The drawing under review shows one solid part. Ordinate dimensions are in mm from its lowest x, y, z. A direction names the side the tool comes from. Give positions to 0.01 mm unless a question says otherwise; leave off trailing zeros. Order: outer loops, then holes, each group sorted by start corner. A loop starts at its lowest first (then second) coordinate and runs counter-clockwise, first axis right, second up. Notation, with made-up numbers: (42, 45.25) -> (46, 45.25) arc R25 ccw to (46, 74.25) -> close; hole circle Ø8 at (52.5, 58.25). An arc over 180 degrees is marked (long way). Use a Markdown table: item, result. Add a question column.
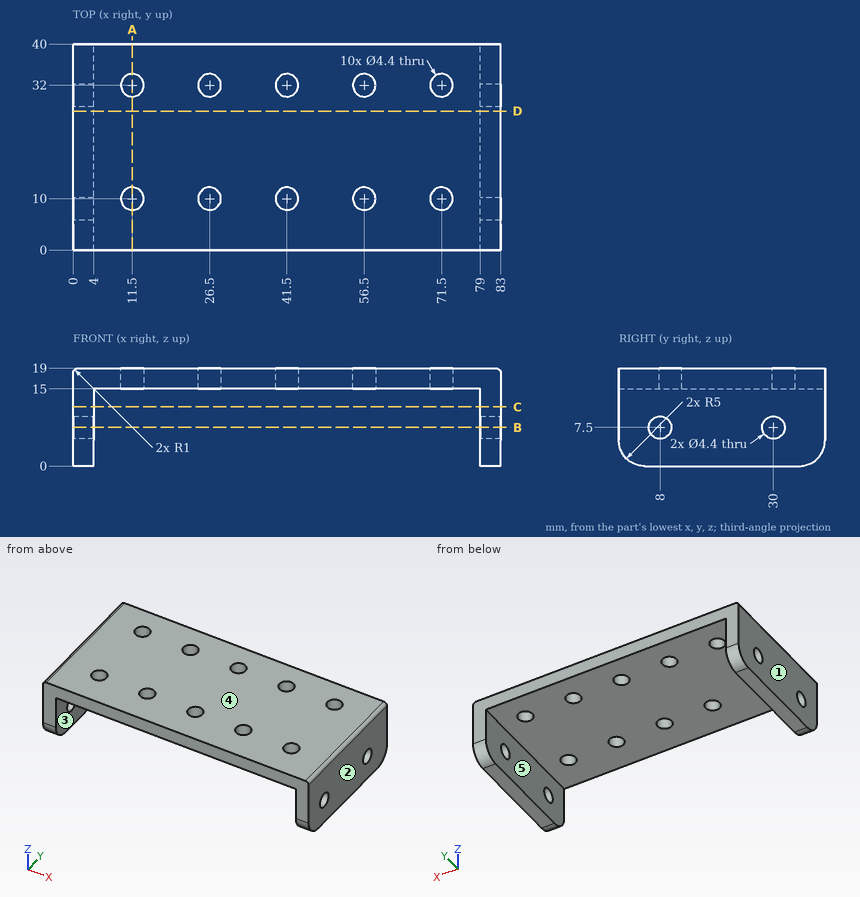
1) For L1, parallel to Y at x = 41.5, z = 17.1; L2, parallel to Y at x = 82.15, z = 7.5; L3, parallel to X at y = 11.5, z = 3.25, list the stretches that pass through material, from the lowest coordinate up. Write a range as [from, to].
2) Add section D-D (y = 27). Give the boundary of the cut face in (x, z).
3) Add section A-A (x = 11.5). Give the boundary of the cut face in (y, z), then the cut area to 3 significant figures.
4) Add section C-C (z = 11.5). Give the boundary of the cut face in (x, y), then the cut area to 3 significant figures.
5) The part is to be moulded in two halves that separate along X. For the marked faces 1, 2 and 3, say which applies: +X half, -X half, draft (parallel to the pull), parting line (faces both ways), or undercut.
6) Machinability: for the marked faces 4 and 5, which of the approach directions +Z, -Z, +X, -X, +Y, -Y give a long, thin tool a straight path to every point of the face, cutting with its end or side? Answer none if there is none.
7) Add section B-B (z = 7.5). Give the boundary of the cut face in (x, y).
8) Insertion check: pin 1 (1.5 mm diameter, centred on x = 37, y = 26, fed in from -Z); pin 2 (4 mm diameter, centred on x = 11.5, y = 32, fed in from -Z); pin 3 (5 mm diameter, centred on y = 30, z = 7.5, fed in from +X). Each pin has a flat end and moves straight along its axis. Give the tip position at first contact, or say it passes through.
Worked answers:
| question | item | result |
|---|---|---|
| 1 | L1 | [0, 7.8], [12.2, 29.8], [34.2, 40] |
| 1 | L2 | [0, 5.8], [10.2, 27.8], [32.2, 40] |
| 1 | L3 | [0, 4], [79, 83] |
| 2 | outline | (0, 0) -> (4, 0) -> (4, 15) -> (79, 15) -> (79, 0) -> (83, 0) -> (83, 18) arc R1 ccw to (82, 19) -> (1, 19) arc R1 ccw to (0, 18) -> close |
| 3 | outline | (0, 15) -> (7.8, 15) -> (7.8, 19) -> (0, 19) -> close; (12.2, 15) -> (29.8, 15) -> (29.8, 19) -> (12.2, 19) -> close; (34.2, 15) -> (40, 15) -> (40, 19) -> (34.2, 19) -> close |
| 3 | area | 125 mm^2 |
| 4 | outline | (0, 0) -> (4, 0) -> (4, 40) -> (0, 40) -> close; (79, 0) -> (83, 0) -> (83, 40) -> (79, 40) -> close |
| 4 | area | 320 mm^2 |
| 5 | face 1 | -X half |
| 5 | face 2 | +X half |
| 5 | face 3 | undercut |
| 6 | face 4 | +Z, +X, -X, +Y, -Y |
| 6 | face 5 | -Z, +Y, -Y |
| 7 | outline | (0, 0) -> (4, 0) -> (4, 5.8) -> (0, 5.8) -> close; (0, 10.2) -> (4, 10.2) -> (4, 27.8) -> (0, 27.8) -> close; (0, 32.2) -> (4, 32.2) -> (4, 40) -> (0, 40) -> close; (79, 0) -> (83, 0) -> (83, 5.8) -> (79, 5.8) -> close; (79, 10.2) -> (83, 10.2) -> (83, 27.8) -> (79, 27.8) -> close; (79, 32.2) -> (83, 32.2) -> (83, 40) -> (79, 40) -> close |
| 8 | pin 1 | z = 15 |
| 8 | pin 2 | through |
| 8 | pin 3 | x = 83 |
